```python
from build123d import *

# Parameters (mm, degrees)
SKETCH1_W                                         = 457.2
SKETCH1_H                                         = 457.2
SKETCH1_R                                         = 50.8
BOSS_EXTRUDE1_DEPTH                               = 6.35
CSK_FOR_6_FLAT_HEAD_MACHINE_SCREW_100_D           = 3.7973
CSK_FOR_6_FLAT_HEAD_MACHINE_SCREW_100_CSINK_D     = 7.0866
CSK_FOR_6_FLAT_HEAD_MACHINE_SCREW_100_CSINK_ANGLE = 100


with BuildPart() as part:
    # Sketch1 → Boss-Extrude1 (new body)
    with BuildSketch(Plane.XY):
        with Locations((228.6, 228.6)):
            Rectangle(SKETCH1_W, SKETCH1_H)
        with Locations((152.4, 228.6)):
            Circle(SKETCH1_R, mode=Mode.SUBTRACT)
    extrude(amount=BOSS_EXTRUDE1_DEPTH)

    # CSK for #6 Flat Head Machine Screw (100)1 (through all)
    with Locations(Plane(origin=(0, 0, 0), x_dir=(-1, 0, 0), z_dir=(0, 0, -1))):
        with Locations((-101.6, 290.195), (-152.4, 290.195), (-203.2, 290.195), (-203.2, 167.005), (-152.4, 167.005), (-101.6, 167.005), (-254, 290.195), (-304.8, 290.195), (-304.8, 167.005), (-254, 167.005)):
            CounterSinkHole(CSK_FOR_6_FLAT_HEAD_MACHINE_SCREW_100_D / 2, CSK_FOR_6_FLAT_HEAD_MACHINE_SCREW_100_CSINK_D / 2, counter_sink_angle=CSK_FOR_6_FLAT_HEAD_MACHINE_SCREW_100_CSINK_ANGLE)


solid = part.part
```
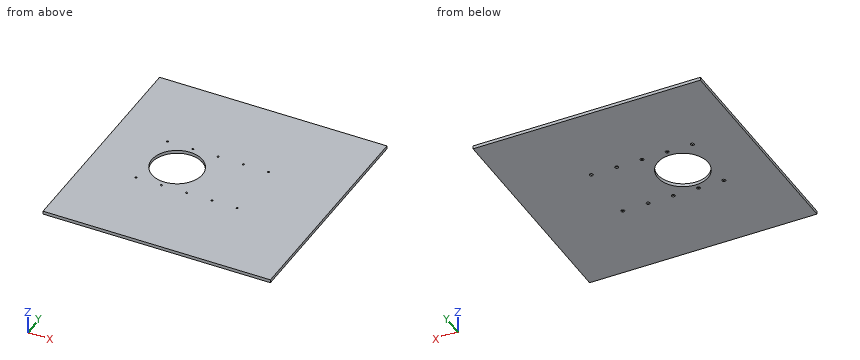
CAD build for the part. Positions are in the model's coordinates, mm. Give positions to 0.01 mm unless a question says otherwise; leave off trailing zeros. Order: outer loops, then holes, each group sorted by start corner. A loop starts at its lowest first (then second) coordinate and runs counter-clockwise, first axis right, second up. Notation, with made-up numbers: M -15.75,54 L -10.75,54 A36 ccw -10.75,92 Z; hole C -34,44.25 d5. An arc over 180 degrees is marked long. Put each result on its own line as item: value. Start each with the question number.
(1) Saw through at A-A, the plane y = 228.6. Write the cut outline in (x, z).
(2) Saw through at B-B, the plane z = 5.25. Give the number of separate pieces and of enclosed holes in the cut face, then the cut area to 3 significant figures.
(3) Drill centre lines: line 1 along Y through (x, z) = (152.4, 4.55); line 2 along Y through (x, z) = (254, 2.55); line 3 along X through (y, z) = (288.5, 3.75). Where is each one in solid material? Low to high.
(4) Flat gauge pin, fed straight in: pin 1 Ø4.5 at (x, y) = (254, 167.005) entering from -Z. Where does the tip first touch, or does it go through?
Check result:
1. outline: M 0,0 L 101.6,0 L 101.6,6.35 L 0,6.35 Z; M 203.2,0 L 457.2,0 L 457.2,6.35 L 203.2,6.35 Z
2. separate pieces: 1
2. enclosed holes: 11
2. area: 201,000 mm2
3. line 1: y = 0 to 165.11, 168.9 to 177.8, 279.4 to 288.3, 292.09 to 457.2
3. line 2: y = 0 to 165.11, 168.9 to 288.3, 292.09 to 457.2
3. line 3: x = 0 to 100.74, 102.46 to 151.54, 153.26 to 202.34, 204.06 to 253.14, 254.86 to 303.94, 305.66 to 457.2
4. pin 1: stops at z = 1.09
